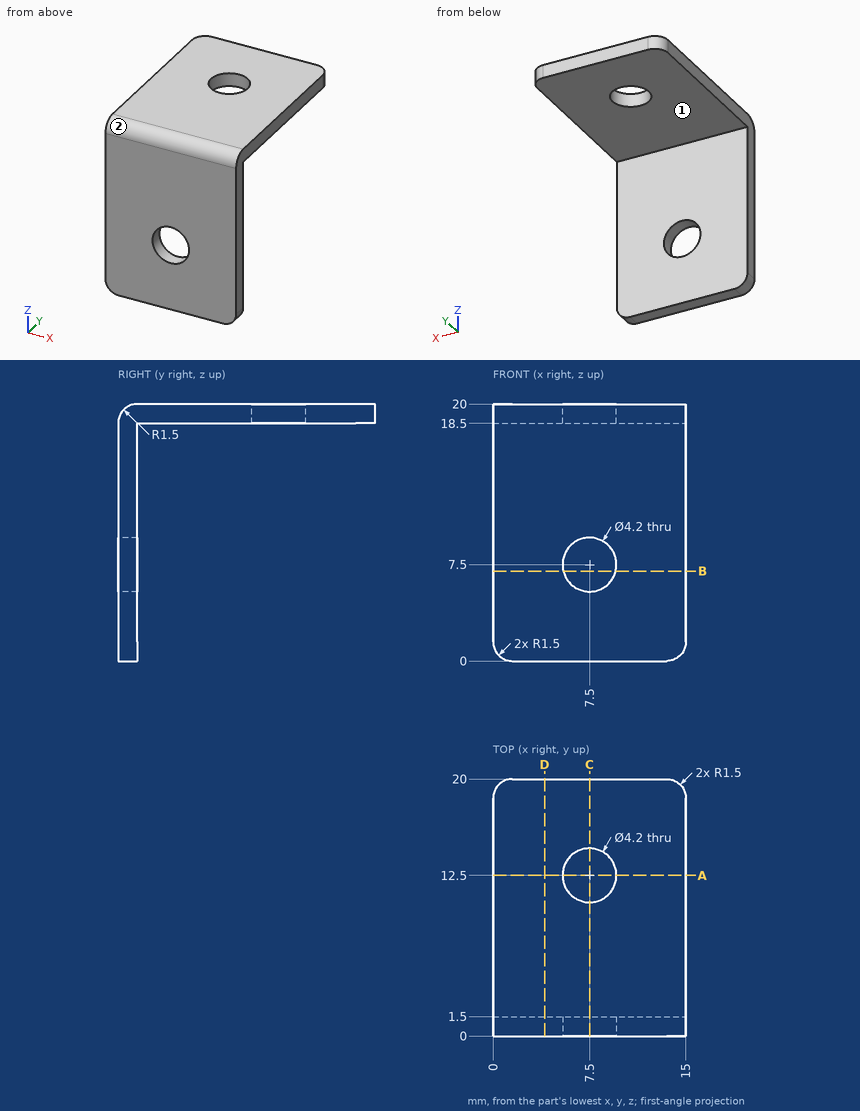
Could you check a few things on this drawing? It's one solid part, dimensions in mm from its lowest x, y, z. A direction names the side the tool comes from. Coordinates: 2 decimals unless noted, no trailing zeros. Order: outer loops, then holes, each group sorted by start corner. A loop starts at its lowest first (then second) coordinate and runs counter-clockwise, first axis right, second up. Notation, with made-up numbers: M 70,6 L 105,6 A26 ccw 105,22 Z; hole C 55.25,61 d6. An arc over 180 degrees is marked long. Answer as a JSON object with one key per item and string values. Group by question number.
(1) Suppose I cut it at C-C, the plane x = 7.5. Please give me the cut outline in (y, z).
(2) For pin 1 (6 mm diameter, centred on x = 1.5, y = 3, fed in from -Z); pin 2 (7.5 mm diameter, centred on x = 5.5, y = 14.5, fed in from -Z); pin 3 (1 mm diameter, centred on x = 11, z = 7, fed in from +Y), each with a flat end and sliding along its axis, tell me the tip position at first contact or that it passes through.
(3) Suppose I cut it at A-A, the plane y = 12.5. Please give me the cut outline in (x, z).
(4) Which directions (+Z, -Z, +X, -X, +Y, -Y) give clear straight access to the entire face, cutting with the end or side of a thin tool? Please do the marked faces 1 and 2.
(5) I need wall thicknesses on probe 1 along X at (y, z) = (0.85, 7.5); probe 2 along Y at (x, z) = (6.25, 5.25); probe 3 along Y at (x, z) = (7.5, 19). Which ranges of each line are inside material? Lowest first, please.
(6) Suppose I cut it at D-D, the plane x = 4. Please give me the cut outline in (y, z), then the cut area to 3 significant figures.
(7) Suppose I cut it at B-B, the plane z = 7. Please give me the cut outline in (x, y), then the cut area to 3 significant figures.
Values found:
{
 "1": {"outline": "M 0,0 L 1.5,0 L 1.5,5.4 L 0,5.4 Z; M 0,9.6 L 1.5,9.6 L 1.5,18.5 L 10.4,18.5 L 10.4,20 L 1.5,20 A1.5 ccw 0,18.5 Z; M 14.6,18.5 L 20,18.5 L 20,20 L 14.6,20 Z"},
 "2": {"pin 1": "stops at z = 0", "pin 2": "stops at z = 18.5", "pin 3": "stops at y = 1.5"},
 "3": {"outline": "M 0,18.5 L 5.4,18.5 L 5.4,20 L 0,20 Z; M 9.6,18.5 L 15,18.5 L 15,20 L 9.6,20 Z"},
 "4": {"face 1": "-Z, +X, -X, +Y", "face 2": "+Z, +X, -X, -Y"},
 "5": {"probe 1": "x = 0 to 5.4, 9.6 to 15", "probe 2": "y = 0 to 1.5", "probe 3": "y = 0.09 to 10.4, 14.6 to 20"},
 "6": {"outline": "M 0,0 L 1.5,0 L 1.5,18.5 L 20,18.5 L 20,20 L 1.5,20 A1.5 ccw 0,18.5 Z", "area": "57.3 mm^2"},
 "7": {"outline": "M 0,0 L 5.46,0 L 5.46,1.5 L 0,1.5 Z; M 9.54,0 L 15,0 L 15,1.5 L 9.54,1.5 Z", "area": "16.4 mm^2"}
}
